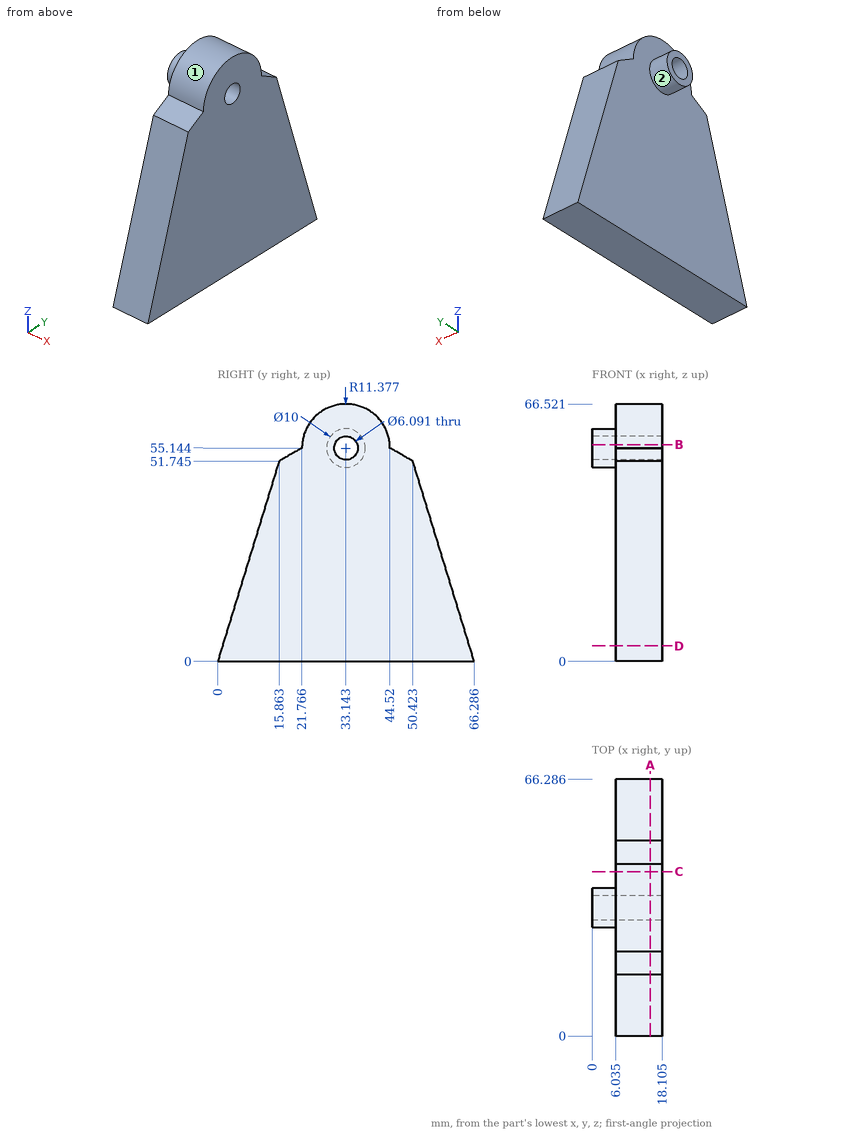
Could you check a few things on this drawing? It's one solid part, dimensions in mm from its lowest x, y, z. A direction names the side the tool comes from. Round coordinates to 2 decimals unless told otherwise and drop trailing zeros. Order: outer loops, then holes, each group sorted by start corner. A loop starts at its lowest first (then second) coordinate and runs counter-clockwise, first axis right, second up. Notation, with made-up numbers: M 38.25,78 L 93.25,78 A21 cw 93.25,92 Z; hole C -5.75,86.5 d1. An arc over 180 degrees is marked long. Use a Markdown table: item, result.
1) Imagine slicing it at D-D (z = 4). List the corners of the cut face in (x, y) for me (1 decimal).
Geometry says:
| item | result |
|---|---|
| outline | M 6,1.2 L 18.1,1.2 L 18.1,65.1 L 6,65.1 Z |
2) If I drill on line 1 along X through (y, z) = (27, 50) (1 decimal); line 2 along Y through (x, z) = (13, 10) (1 decimal); line 3 along Y through (x, z) = (9, 17.5) (1 decimal), over which ranges is the centre line in solid material (lowest first)?
Geometry says:
| item | result |
|---|---|
| line 1 | x = 6 to 18.1 |
| line 2 | y = 3.1 to 63.2 |
| line 3 | y = 5.4 to 60.9 |
3) On a 3-axis mill with a long thin cutter (end or side, diameter ignored), from which of +Z, -Z, +X, -X, +Y, -Y can I reach the whole of each face in a straight line? I mean the marked faces 1 and 2. Say none if no direction works.
Geometry says:
| item | result |
|---|---|
| face 1 | +Z, +X, -X |
| face 2 | -X |
4) I'm going to push flat-ended pins straight in: P1, Ø1.5, axis at x = 15, y = 37.5, coming from the +Z side (1 decimal); P2, Ø6, axis at y = 41.5, z = 11, coming from the -X side (3 decimals). Where does each tip first touch, or does it pass through?
Geometry says:
| item | result |
|---|---|
| P1 | stops at z = 65.9 |
| P2 | stops at x = 6.035 |
5) Imagine slicing it at C-C (y = 42.5). List the corners of the cut face in (x, z) for me (1 decimal), then the cut area to 3 significant figures.
Geometry says:
| item | result |
|---|---|
| outline | M 6,0 L 18.1,0 L 18.1,61.6 L 6,61.6 Z |
| area | 744 mm² |
6) Imagine slicing it at A-A (x = 15). List the corners of the cut face in (y, z) for me (1 decimal).
Geometry says:
| item | result |
|---|---|
| outline | M 0,0 L 66.3,0 L 50.4,51.7 L 44.5,55.1 A11.4 ccw 21.8,55.1 L 15.9,51.7 Z; hole C 33.1,55.1 d6.1 |
7) Imagine slicing it at B-B (z = 56). List the corners of the cut face in (x, y) for me (1 decimal).
Geometry says:
| item | result |
|---|---|
| outline | M 0,28.2 L 6,28.2 L 6,21.8 L 18.1,21.8 L 18.1,30.2 L 0,30.2 Z; M 0,36.1 L 18.1,36.1 L 18.1,44.5 L 6,44.5 L 6,38.1 L 0,38.1 Z |
